Geometry: see drawing. Coordinates: mm, zero at the bounding-box minimum. A direction names the side the tool comes from. Round coordinates to 2 decimals unless told otherwise and drop trailing zeros. Order: outer loops, then holes, each group sorted by start corner. A loop starts at its lowest first (then second) coordinate and runs counter-clockwise, first axis right, second up. Notation, with made-up numbers: (74, -29.75) -> (118, -29.75) arc R11 ccw to (118, -17.75) -> close; hole circle Ø8 at (59.5, 75). An arc over 180 degrees is marked (long way). Put each result on its own line as item: value.
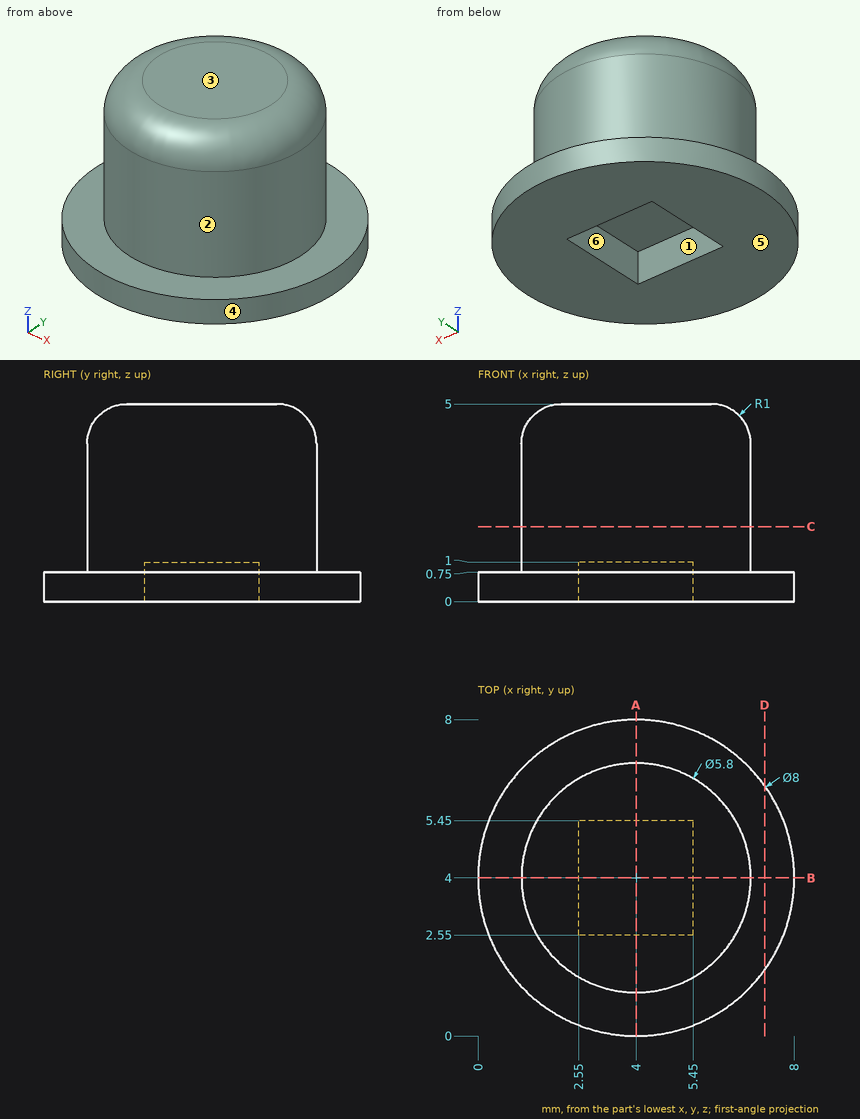
1. Material intervals for probe 1 along Z at (x, y) = (0.5, 4.5); probe 2 along Z at (x, y) = (4.5, 3.25); probe 3 along Y at (x, z) = (4, 2.4), sorted ascending.
Ans:
probe 1: 0 to 0.75
probe 2: 1 to 5
probe 3: 1.1 to 6.9
2. Cut plane A-A on x = 4. Return loops of the section in (y, z), and give its area (3 significant figures).
Ans:
outline: (0, 0) -> (2.55, 0) -> (2.55, 1) -> (5.45, 1) -> (5.45, 0) -> (8, 0) -> (8, 0.75) -> (6.9, 0.75) -> (6.9, 4) arc R1 ccw to (5.9, 5) -> (2.1, 5) arc R1 ccw to (1.1, 4) -> (1.1, 0.75) -> (0, 0.75) -> close
area: 27.3 mm²
3. Draft query along X for the marked faces 4, 5 and 6. Return one class per face: +X half, -X half, draft (parallel to the pull), parting line (faces both ways), or undercut.
Ans:
face 4: parting line
face 5: draft
face 6: undercut
4. Cut plane D-D on x = 7.25. Return loops of the section in (y, z).
Ans:
outline: (1.67, 0) -> (6.33, 0) -> (6.33, 0.75) -> (1.67, 0.75) -> close
5. Set-up query: the marked faces 1, 2 and 3. Return all of +Z, -Z, +X, -X, +Y, -Y with unobstructed straight access to the full face (end or side cutting, diameter ignored); none if empty.
Ans:
face 1: -Z
face 2: +Z
face 3: +Z, +X, -X, +Y, -Y
6. Contact query for flat-ended pins moving along their axis: P1, Ø1, axis at x = 1, z = 1, coming from the +Y side; P2, Ø2, axis at x = 6.5, z = 1.5, coming from the +Y side; P3, Ø1.5, axis at x = 3.5, y = 4.5, coming from the -Z side. Output: stop coordinate, or through.
Ans:
P1: y = 7.07
P2: y = 7.55
P3: z = 1
7. Cut plane C-C on z = 1.9. Return loops of the section in (x, y), and give its area (3 significant figures).
Ans:
outline: circle Ø5.8 at (4, 4)
area: 26.4 mm²
